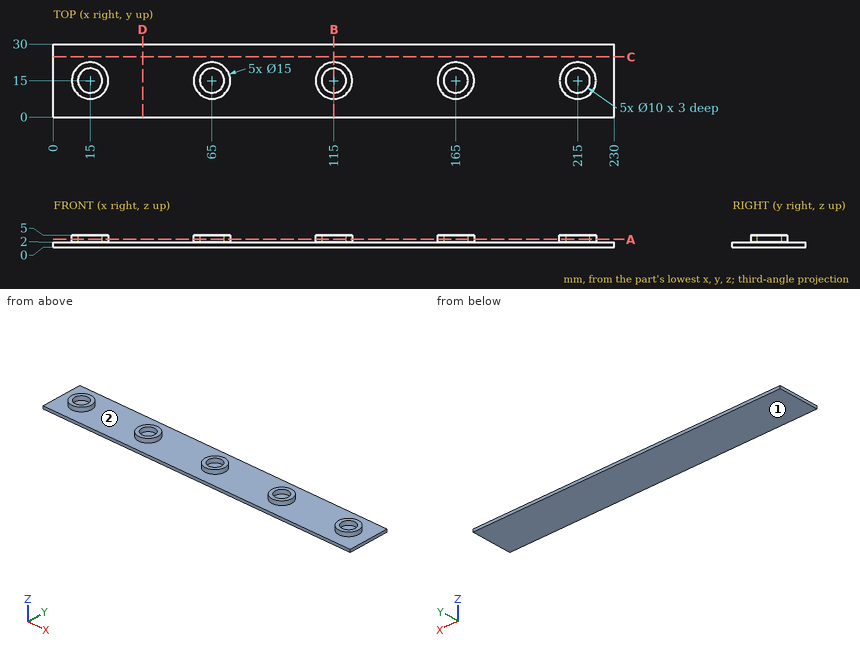
Drawing for the job (mm, zero at the part's lowest x, y, z). Coordinates: 2 decimals unless noted, no trailing zeros. Order: outer loops, then holes, each group sorted by start corner. A loop starts at its lowest first (then second) coordinate and runs counter-clockwise, first axis right, second up. Notation, with made-up numbers: (42.25, -6.75) -> (86.25, -6.75) arc R16 cw to (86.25, 18.25) -> close; hole circle Ø10 at (15.25, 88). An arc over 180 degrees is marked (long way). Return JSON: item names as keys, results as strings.
Item 1: Slice it at B-B (x = 115). Write the cut outline in (y, z).
Model answer:
{"outline": "(0, 0) -> (30, 0) -> (30, 2) -> (22.5, 2) -> (22.5, 5) -> (20, 5) -> (20, 2) -> (10, 2) -> (10, 5) -> (7.5, 5) -> (7.5, 2) -> (0, 2) -> close"}
Item 2: Slice it at A-A (z = 3.25). Count the separate pieces of the cut face and the enclosed holes in it, then the cut area to 3 significant figures.
Model answer:
{"separate pieces": "5", "enclosed holes": "5", "area": "491 mm²"}
Item 3: Wall check: line 1 along Y through (x, z) = (15, 3.75); line 2 along Z through (x, y) = (148.5, 27.5); line 3 along Y through (x, z) = (160.5, 2.9). Give the ranges that are in metal, low to high. Write a range as from..to.
Model answer:
{"line 1": "y = 7.5..10, 20..22.5", "line 2": "z = 0..2", "line 3": "y = 9..12.82, 17.18..21"}
Item 4: Slice it at D-D (x = 36.5). Write the cut outline in (y, z).
Model answer:
{"outline": "(0, 0) -> (30, 0) -> (30, 2) -> (0, 2) -> close"}
Item 5: Mould opens along X. For the marked faces 1 and 2 say: pulls with the +X half, pulls with the -X half, needs draft (parallel to the pull), parting line crosses it, or undercut.
Model answer:
{"face 1": "needs draft", "face 2": "undercut"}
Item 6: Pin check, flat tips, straight feed: P1, Ø8, axis at x = 162.5, y = 15, coming from the +Z side; P2, Ø3, axis at x = 16.5, y = 16.5, coming from the +Z side. Stop position of each tip, or through.
Model answer:
{"P1": "stops at z = 5", "P2": "stops at z = 2"}
Item 7: Slice it at C-C (y = 24.75). Write the cut outline in (x, z), then the cut area to 3 significant figures.
Model answer:
{"outline": "(0, 0) -> (230, 0) -> (230, 2) -> (0, 2) -> close", "area": "460 mm²"}
